Geometry check sheet. Reference: the model listing, model coordinates, mm. A direction names the side the tool comes from. Coordinates: 2 decimals unless noted, no trailing zeros. Loops run counter-clockwise (first coordinate to the right, second up) from the corner with the lowest first, then second, coordinate; pieces in that order, holes last.
from build123d import *

# Parameters (mm, degrees)
F0_R     = 9
F1_DEPTH = 150
F3_DEPTH = 13.5


with BuildPart() as f1:
    # F0 (on Right) → F1 (new body)
    with BuildSketch(Plane.YZ):
        Circle(F0_R)
    extrude(amount=F1_DEPTH)

    # F2 (on face) → F3 (join)
    with BuildSketch(Plane.YZ.offset(150)):
        Polygon((-16.301647, 2.23748), (-10.088538, -12.9989), (6.213108, -15.23638), (16.301647, -2.23748), (10.088538, 12.9989), (-6.213108, 15.23638), align=None)
    extrude(amount=-F3_DEPTH)


solid = f1.part
(1) Sectioned sample at D-D on z = -11.5. Record the cut outline in (x, y).
Findings:
outline: (136.5, -10.7) - (150, -10.7) - (150, 9.11) - (136.5, 9.11) - close
(2) Sectioned sample at C-C on x = 31.5. Record the cut outline in (y, z).
Findings:
outline: circle Ø18 at (0, 0)
(3) Scan lines: L1, parallel to X at y = 12, z = -1; L2, parallel to Z at x = 56, y = 6. Record each from-to range of solid material in increasing order.
Findings:
L1: x = 136.5 to 150
L2: z = -6.71 to 6.71
(4) Access from +Z, -Z, +X, -X, +Y, -Y to the whole of each face (thin tool, end or side, straight path). Record for faces 1 (the cylindrical face through (67.294, -1.172, 8.923)), 2 (the flat face through (143.34, 13.24, 5.27)).
Findings:
face 1: -X
face 2: +Z, +X, -X, +Y
(5) Sectioned sample at B-B on z = 7.5. Record the cut outline in (x, y).
Findings:
outline: (0, -4.97) - (136.5, -4.97) - (136.5, -12.22) - (150, -12.22) - (150, 12.33) - (136.5, 12.33) - (136.5, 4.97) - (0, 4.97) - close
(6) Gauge pin test, flat ends, axial feed: pin 1 Ø2 at (x, y) = (67, 3) entering from +Z; pin 2 Ø12 at (x, z) = (37.5, -6.5) entering from -Y; pin 3 Ø4 at (x, z) = (37.5, 0) entering from +Y. Record the tip position at first contact, or that the pin passes through.
Findings:
pin 1: stops at z = 8.77
pin 2: stops at y = -8.99
pin 3: stops at y = 9
(7) Sectioned sample at A-A on y = 0. Record the cut outline in (x, z), and give its area (3 significant figures).
Findings:
outline: (0, -9) - (136.5, -9) - (136.5, -14.38) - (150, -14.38) - (150, 14.38) - (136.5, 14.38) - (136.5, 9) - (0, 9) - close
area: 2,850 mm2
